Build history of the part. All positions in model axes, mm. A direction names the side the tool comes from. Give positions to 0.01 mm unless a question says otherwise; leave off trailing zeros. Loops run counter-clockwise (first coordinate to the right, second up) from the corner with the lowest first, then second, coordinate; pieces in that order, holes last. Notation, with made-up numbers: M -26.5,72 L -16.5,72 A7 cw -16.5,78 Z; hole C 79.5,63.25 d2. An arc over 180 degrees is marked long. Answer as a JSON object with one key per item and string values. Group by question number.
1. Slice it at B-B (y = -17). List the corners of the cut face in (x, z), then the cut area to 3 significant figures.
2. Slice it at A-A (z = 40). List the corners of the cut face in (x, y), then the cut area to 3 significant figures.
3. Drop flat-ended pins along their axis: pin 1 Ø12 at (x, z) = (-113, 36.5) entering from +Y; pin 2 Ø10 at (x, y) = (-48, -68) entering from +Z; pin 3 Ø1 at (y, z) = (-102.5, 21) entering from -X. Give the stop position or say it passes through.
4. Slice it at C-C (x = -25.5). List the corners of the cut face in (y, z), then the cut area to 3 significant figures.
5. Slice it at D-D (z = 54). List the corners of the cut face in (x, y).
6. 3-axis set-ups, long thin cutter, end or side, ignore diameter. For faces 1 (the face through (-148.028, -99.02, 8.085)), 2 (the face through (-4, -59, 32)), 3 (the face through (-1.97, -107.58, 28.49)): which of +Z, -Z, +X, -X, +Y, -Y reach the whole face in a straight line?
7. Drill centre lines: line 1 along X through (y, z) = (-110, 16); line 2 along Y through (x, z) = (-73, 48.5); line 3 along Y through (x, z) = (-7.5, 57). Where is each one in solid material? Low to high. Write a range as [from, to].
8. Mould opens along X. For faces 4 (the face through (-148, -97, 15.447)), 5 (the face through (0, -61, 30)), 6 (the face through (-150, -61, 30)), 7 (the face through (-76, -2, 2)) say: released by +X, released by -X, zero draft, split by the parting line, or undercut.
from build123d import *

# Parameters (mm, degrees)
F0_W      = 120
F0_H      = 60
F0_R      = 6
F1_DEPTH  = 150
F2_W      = 142
F2_H      = 116
F3_DEPTH  = 56
F4_W      = 5
F4_H      = 56
F5_DEPTH  = 2
F6_W      = 5
F6_H      = 56
F7_DEPTH  = 2
F9_DEPTH  = 2
F10_R     = 2.25
F11_DEPTH = 11.6
F10_W     = 19
F10_H     = 28
F12_DEPTH = 25
F13_DEPTH = 25
F15_DEPTH = 20
F14_W     = 5
F14_H     = 5
F16_DEPTH = 56


with BuildPart() as f1:
    # F0 (on Right) → F1 (new body)
    with BuildSketch(Plane.YZ):
        with Locations((-60, 30)):
            Rectangle(F0_W, F0_H)
        with Locations((-102.817491, 32.142658)):
            Circle(F0_R, mode=Mode.SUBTRACT)
        with Locations((-102.817491, 32.142658)):
            Circle(F0_R)
    extrude(amount=-F1_DEPTH)

    # F2 (on face) → F3 (cut)
    with BuildSketch(Plane.XY.offset(60)):
        with Locations((-75, -58)):
            Rectangle(F2_W, F2_H)
    extrude(amount=-F3_DEPTH, mode=Mode.SUBTRACT)

    # F4 (on face) → F5 (cut)
    with BuildSketch(Plane(origin=(-4, 0, 0), x_dir=(0, -1, 0), z_dir=(-1, 0, 0))):
        with Locations((2.5, 32)):
            Rectangle(F4_W, F4_H)
    extrude(amount=-F5_DEPTH, mode=Mode.SUBTRACT)

    # F6 (on face) → F7 (cut)
    with BuildSketch(Plane.YZ.offset(-146)):
        with Locations((-2.5, 32)):
            Rectangle(F6_W, F6_H)
    extrude(amount=-F7_DEPTH, mode=Mode.SUBTRACT)

    # F8 (on face) → F9 (cut)
    with BuildSketch(Plane.XY.offset(4)):
        Polygon((-4, -5), (-2, -5), (-2, 0), (-148, 0), (-148, -5), (-146, -5), align=None)
    extrude(amount=-F9_DEPTH, mode=Mode.SUBTRACT)

    # F10 (on face) → F11 (cut)
    with BuildSketch(Plane(origin=(-150, 0, 0), x_dir=(0, -1, 0), z_dir=(-1, 0, 0))):
        with Locations((96.941963, 49.947112)):
            Circle(F10_R)
    extrude(amount=-F11_DEPTH, mode=Mode.SUBTRACT)

    # F10 (on face) → F12 (cut)
    with BuildSketch(Plane(origin=(-150, 0, 0), x_dir=(0, -1, 0), z_dir=(-1, 0, 0))):
        with Locations((96.941963, 29.447112)):
            Rectangle(F10_W, F10_H)
    extrude(amount=-F12_DEPTH, mode=Mode.SUBTRACT)

    # F10 (on face) → F13 (cut)
    with BuildSketch(Plane(origin=(-150, 0, 0), x_dir=(0, -1, 0), z_dir=(-1, 0, 0))):
        with Locations((96.941963, 8.947112)):
            Circle(F10_R)
    extrude(amount=-F13_DEPTH, mode=Mode.SUBTRACT)

    # F0 (on Right) → F15 (cut)
    with BuildSketch(Plane.YZ):
        with Locations((-102.817491, 32.142658)):
            Circle(F0_R)
    extrude(amount=-F15_DEPTH, mode=Mode.SUBTRACT)

    # F14 (on face) → F16 (join)
    with BuildSketch(Plane.XY.offset(4)):
        with Locations((-6.5, -113.5)):
            Rectangle(F14_W, F14_H)
        with Locations((-143.5, -113.5)):
            Rectangle(F14_W, F14_H)
    extrude(amount=F16_DEPTH)


solid = f1.part
Established:
{
 "1": {"outline": "M -150,0 L 0,0 L 0,60 L -4,60 L -4,4 L -146,4 L -146,60 L -150,60 Z", "area": "1,050 mm^2"},
 "2": {"outline": "M -150,-120 L 0,-120 L 0,0 L -2,0 L -2,-5 L -4,-5 L -4,-111 L -9,-111 L -9,-116 L -141,-116 L -141,-111 L -146,-111 L -146,-106.44 L -150,-106.44 Z; M -150,-87.44 L -146,-87.44 L -146,-5 L -148,-5 L -148,0 L -150,0 Z", "area": "1,480 mm^2"},
 "3": {"pin 1": "stops at y = -116", "pin 2": "stops at z = 4", "pin 3": "stops at x = -4"},
 "4": {"outline": "M -120,0 L 0,0 L 0,2 L -5,2 L -5,4 L -116,4 L -116,60 L -120,60 Z", "area": "694 mm^2"},
 "5": {"outline": "M -150,-120 L 0,-120 L 0,0 L -2,0 L -2,-5 L -4,-5 L -4,-111 L -9,-111 L -9,-116 L -141,-116 L -141,-111 L -146,-111 L -146,-5 L -148,-5 L -148,0 L -150,0 Z"},
 "6": {"face 1": "-X", "face 2": "+Z, +Y", "face 3": "+X"},
 "7": {"line 1": "x = [-150, -146], [-4, 0]", "line 2": "y = [-120, -116]", "line 3": "y = [-120, -111]"},
 "8": {"face 4": "zero draft", "face 5": "released by +X", "face 6": "released by -X", "face 7": "undercut"}
}
